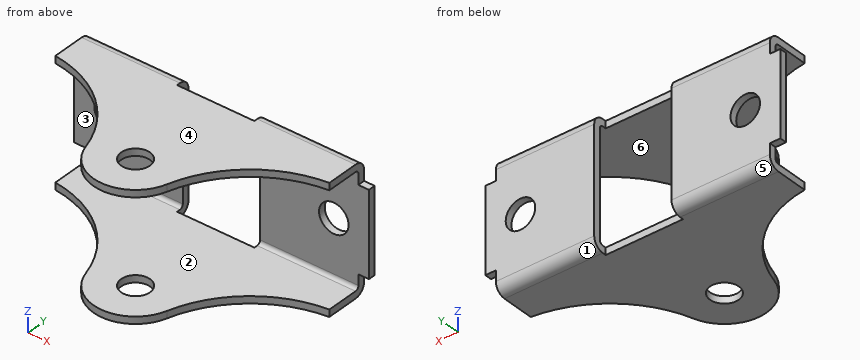
```python
from build123d import *

# Parameters (mm, degrees)
SKETCH_1_R                       = 2.05
SM_BASE_FLANGE_2_DEPTH           = 1
SM_EDGE_FLANGE_1_STRIP_W         = 5
SM_EDGE_FLANGE_1_STRIP_H         = 1
SM_EDGE_FLANGE_1_STRIP_CUT_DEPTH = 42
SM_EDGE_FLANGE_1_DEPTH           = 42
SKETCH_13_W                      = 11
SKETCH_13_H                      = 2
CUT_EXTRUDE_1_DEPTH              = 35.727510708
SKETCH_14_R                      = 2.1
SKETCH_14_W                      = 1.5
SKETCH_14_H                      = 3
CUT_EXTRUDE_2_DEPTH              = 36.341194094


# Sheet-metal steps are written as plain solids
with BuildPart() as part:
    # Sketch 1 → Базовая кромка2 (new body)
    with BuildSketch(Plane.XY):
        with BuildLine():
            Line((-21, -5), (-21, 0))
            Line((-21, 0), (21, 0))
            Line((21, 0), (21, -5))
            ThreePointArc((21, -5), (11.451449282, -8.286050683), (5.772615091, -16.636128055))
            ThreePointArc((5.772615091, -16.636128055), (0, -21), (-5.772615091, -16.636128055))
            ThreePointArc((-5.772615091, -16.636128055), (-11.451449282, -8.286050683), (-21, -5))
        make_face()
        with Locations((0, -15)):
            Circle(SKETCH_1_R, mode=Mode.SUBTRACT)
    extrude(amount=-SM_BASE_FLANGE_2_DEPTH)

    # Ребро-кромка1 strip (across the edge) → Ребро-кромка1 strip cut (cut)
    with BuildSketch(Plane(origin=(-21, 0, -1), x_dir=(0, -1, 0), z_dir=(1, 0, 0))):
        with Locations((-2, -0.5)):
            Rectangle(SM_EDGE_FLANGE_1_STRIP_W, SM_EDGE_FLANGE_1_STRIP_H)
    extrude(amount=SM_EDGE_FLANGE_1_STRIP_CUT_DEPTH, mode=Mode.SUBTRACT)

    # Ребро-кромка1 section (across the edge) → Ребро-кромка1 (add)
    with BuildSketch(Plane(origin=(-21, 0, -1), x_dir=(0, -1, 0), z_dir=(1, 0, 0))):
        with BuildLine():
            Line((-1, 0.5), (-1, 8))
            Line((-1, 8), (0, 8))
            Line((0, 8), (0, 0.5))
            ThreePointArc((0, 0.5), (0.146446609, 0.146446609), (0.5, 0))
            Line((0.5, 0), (0.5, -1))
            ThreePointArc((0.5, -1), (-0.560660172, -0.560660172), (-1, 0.5))
        make_face()
    extrude(amount=SM_EDGE_FLANGE_1_DEPTH)

    # Зеркальное отражение1: part across plane


with BuildPart() as part_1:
    add(part.part)
    add(part.part.mirror(Plane(origin=(-21, 1, -9), x_dir=(1, 0, 0), z_dir=(0, 0, 1))))

    # Эскиз13 → Вырез-Вытянуть1 (cut, through all)
    with BuildSketch(Plane.XY):
        Rectangle(SKETCH_13_W, SKETCH_13_H)
    extrude(amount=-CUT_EXTRUDE_1_DEPTH, mode=Mode.SUBTRACT)

    # Эскиз14 → Вырез-Вытянуть2 (cut, through all)
    with BuildSketch(Plane(origin=(0, 1, 0), x_dir=(1, 0, 0), z_dir=(0, 1, 0))):
        with Locations(Location((-16, 9, 0), (0, 0, 90))):
            Circle(SKETCH_14_R)
        with Locations(Location((16, 9, 0), (0, 0, 90))):
            Circle(SKETCH_14_R)
        with Locations((-20.25, 16.5)):
            Rectangle(SKETCH_14_W, SKETCH_14_H)
        with Locations((-20.25, 1.5)):
            Rectangle(SKETCH_14_W, SKETCH_14_H)
        with Locations((20.25, 1.5)):
            Rectangle(SKETCH_14_W, SKETCH_14_H)
        with Locations((20.25, 16.5)):
            Rectangle(SKETCH_14_W, SKETCH_14_H)
    extrude(amount=-CUT_EXTRUDE_2_DEPTH, mode=Mode.SUBTRACT)


solid = part_1.part
```
For this review, take the finished solid that the model builds, in its own axes (mm). Face numbers are marked on the shaded views. A direction names the side the tool comes from. Round coordinates to 2 decimals unless told otherwise and drop trailing zeros. Write each loop counter-clockwise with the first axis right and the second up, starting at its lowest first coordinate (ties: lowest second). Pieces come first, ordered by that corner, then holes.
1) Machinability: for the marked faces 5 and 6, which of the approach directions +Z, -Z, +X, -X, +Y, -Y give a long, thin tool a straight path to every point of the face, cutting with its end or side? Answer none if there is none.
Answer below:
face 5: -Z, +X, -X, +Y
face 6: +X, -X, -Y
2) Mouldability with a two-part tool opening along Z and no side actions: class the marked faces 1, 2, 3 and 4 as +Z half, -Z half, draft (parallel to the pull), parting line (faces both ways), or undercut.
Answer below:
face 1: -Z half
face 2: undercut
face 3: undercut
face 4: +Z half
3) Take a section at B-B on x = 0. Give the boundary of the cut face in (y, z), then the cut area to 3 significant figures.
Answer below:
outline: (-21, -18) - (-17.05, -18) - (-17.05, -17) - (-21, -17) - close; (-21, -1) - (-17.05, -1) - (-17.05, 0) - (-21, 0) - close; (-12.95, -18) - (-1, -18) - (-1, -17) - (-12.95, -17) - close; (-12.95, -1) - (-1, -1) - (-1, 0) - (-12.95, 0) - close
area: 31.8 mm2
4) Take a section at C-C on z = -9. Give the boundary of the cut face in (x, y).
Answer below:
outline: (-21, 0) - (-18.1, 0) - (-18.1, 1) - (-21, 1) - close; (-13.9, 0) - (-5.5, 0) - (-5.5, 1) - (-13.9, 1) - close; (5.5, 0) - (13.9, 0) - (13.9, 1) - (5.5, 1) - close; (18.1, 0) - (21, 0) - (21, 1) - (18.1, 1) - close
5) For line 1 along X through (y, z) = (0.4, -9); line 2 along Y through (x, z) = (0, -0.6); line 3 along Z through (x, y) = (4.5, -11.5), list the stretches that pass through material, from the lowest coordinate up.
Answer below:
line 1: x = -21 to -18.1, -13.9 to -5.5, 5.5 to 13.9, 18.1 to 21
line 2: y = -21 to -17.05, -12.95 to -1
line 3: z = -18 to -17, -1 to 0
6) Insertion check: pin 1 Ø1.1 at (x, y) = (20.5, 0.5) entering from -Z; pin 2 Ø0.5 at (x, y) = (-20.5, 0.5) entering from +Z; pin 3 Ø10 at (x, y) = (-5.5, -10) entering from +Z; pin 4 Ø3.5 at (x, y) = (0, -15) entering from +Z. Each pin has a flat end and moves straight along its axis. Give the tip position at first contact, or say it passes through.
Answer below:
pin 1: stops at z = -15
pin 2: stops at z = -3
pin 3: stops at z = 0
pin 4: passes through
7) Take a section at A-A on y = -2.25. Give the boundary of the cut face in (x, z).
Answer below:
outline: (-19.5, -18) - (19.5, -18) - (19.5, -17) - (-19.5, -17) - close; (-19.5, -1) - (19.5, -1) - (19.5, 0) - (-19.5, 0) - close
8) Take a section at D-D on z = -5.5. Give the boundary of the cut face in (x, y).
Answer below:
outline: (-21, 0) - (-5.5, 0) - (-5.5, 1) - (-21, 1) - close; (5.5, 0) - (21, 0) - (21, 1) - (5.5, 1) - close
